```python
from build123d import *

# Parameters (mm, degrees)
CROQUIS1_R              = 12.7
SALIENTE_EXTRUIR1_DEPTH = 740
CROQUIS2_W              = 0.777166432
CROQUIS2_H              = 0.57610026
SALIENTE_EXTRUIR2_DEPTH = 10
CROQUIS3_R              = 12


with BuildPart() as part:
    # Croquis1 → Saliente-Extruir1 (new body)
    with BuildSketch(Plane.XY):
        Circle(CROQUIS1_R)
    extrude(amount=SALIENTE_EXTRUIR1_DEPTH)

    # Croquis2 → Saliente-Extruir2 (add)
    with BuildSketch(Plane.XY.offset(740)):
        with Locations((0, 12.7)):
            Rectangle(CROQUIS2_W, CROQUIS2_H)
    extrude(amount=-SALIENTE_EXTRUIR2_DEPTH)

    # Barrer1: sweep along a curve in space
    with BuildLine() as barrer1_path:
        Line((0, 0, 740), (0, 0, 800))
        Line((0, 0, 800), (-200, 0, 800))
    # Croquis3 → Barrer1 (sweep)
    with BuildSketch(Plane.XY.offset(740)):
        Circle(CROQUIS3_R)
    sweep(path=barrer1_path.line, transition=Transition.RIGHT)


solid = part.part
```
Input: part model. Units: mm. Frame: model coordinates. A direction names the side the tool comes from. Give positions to 0.01 mm unless a question says otherwise; leave off trailing zeros. Loops run counter-clockwise (first coordinate to the right, second up) from the corner with the lowest first, then second, coordinate; pieces in that order, holes last.
1) Reachability of faces 4 (the cylindrical face through (-2.75, -12.4, 364.82)), 5 (the flat face through (-0.1, -12.2, 740)), 6 (the flat face through (0, 0, 0)) from +Z, -Z, +X, -X, +Y, -Y: full face, straight path, thin tool, end or side. Return the list, or none.
A:
face 4: -Z
face 5: none
face 6: -Z, +X, -X, +Y, -Y
2) Section query C-C on z = 175. Return the cut outline in (x, y), and give its area (3 significant figures).
A:
outline: circle Ø25.4 at (0, 0)
area: 507 mm2
3) Section query A-A on y = 0. Return the cut outline in (x, z), and give its area (3 significant figures).
A:
outline: (-200, 788) - (-12, 788) - (-12, 740) - (-12.7, 740) - (-12.7, 0) - (12.7, 0) - (12.7, 740) - (12, 740) - (12, 812) - (-200, 812) - close
area: 25,000 mm2
4) Section query D-D on z = 800. Return the cut outline in (x, y), and give its area (3 significant figures).
A:
outline: (-200, -12) - (0, -12) arc R12 ccw to (0, 12) - (-200, 12) - close
area: 5,030 mm2
5) Section query B-B on x = -48.5. Return the cut outline in (y, z).
A:
outline: circle Ø24 at (0, 800)
6) Mould query, pull axis Z, two halves, no side actions, for faces 1 (the cylindrical face through (-95.484, 3.604, 811.446)), 2 (the flat face through (-200, 0, 800)), 3 (the cylindrical face through (11.085, -4.596, 768.504)). Classes: released by +Z, released by -Z, zero draft, split by the parting line, or undercut.
A:
face 1: split by the parting line
face 2: zero draft
face 3: undercut
7) Contact query for flat-ended pins moving along their axis: pin 1 (3 mm diameter, centred on x = -10.5, z = 450, fed in from -Y); pin 2 (5 mm diameter, centred on y = 5, z = 347, fed in from +X); pin 3 (4 mm diameter, centred on y = -7.5, z = 212, fed in from -X). Output: stop coordinate, or through.
A:
pin 1: stops at y = -8.96
pin 2: stops at x = 12.45
pin 3: stops at x = -11.45
8) Line query: L1, parallel to Y at x = -0.5, z = 353; L2, parallel to X at y = -1.5, z = 432.5; L3, parallel to Z at x = -1, y = -1.5. Output: solid intervals per line, ascending.
A:
L1: y = -12.69 to 12.69
L2: x = -12.61 to 12.61
L3: z = 0 to 811.91
